The model under review builds one solid part; all positions refer to its coordinate system, in mm. Face numbers are marked on the shaded views. A direction names the side the tool comes from. Coordinates: 2 decimals unless noted, no trailing zeros. Write each loop counter-clockwise with the first axis right and the second up, starting at its lowest first coordinate (ties: lowest second). Pieces come first, ordered by that corner, then holes. Notation, with made-up numbers: (79.5, -37.5) -> (109.5, -37.5) arc R16 ccw to (109.5, -24.5) -> close; hole circle Ø4 at (14.5, 6). An arc over 180 degrees is marked (long way). Write each question's results on one line, items separated by ' | '.
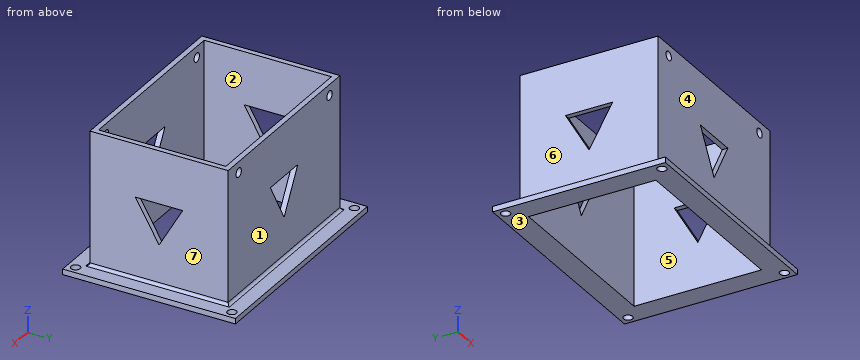
```python
from build123d import *

# Parameters (mm, degrees)
SKETCH_1_W          = 125
SKETCH_1_H          = 95
SKETCH_1_W_2        = 100
SKETCH_1_H_2        = 70
EXTRUDE_1_DEPTH     = 3
SKETCH_2_W          = 106
SKETCH_2_H          = 76
SKETCH_2_W_2        = 100
SKETCH_2_H_2        = 70
EXTRUDE_2_DEPTH     = 73.5
SKETCH_3_R          = 2.5
CUT_EXTRUDE_1_DEPTH = 113.5
FILLET_1_R          = 1.5
SKETCH_4_R          = 2.5
CUT_EXTRUDE_2_DEPTH = 113.5
CUT_EXTRUDE_3_DEPTH = 113.5
CUT_EXTRUDE_4_DEPTH = 113.5


with BuildPart() as part:
    # 草图1 → 凸台-拉伸1 (new body)
    with BuildSketch(Plane.XY):
        Rectangle(SKETCH_1_W, SKETCH_1_H)
        Rectangle(SKETCH_1_W_2, SKETCH_1_H_2, mode=Mode.SUBTRACT)
    extrude(amount=EXTRUDE_1_DEPTH)

    # 草图2 → 凸台-拉伸2 (add)
    with BuildSketch(Plane.XY.offset(3)):
        Rectangle(SKETCH_2_W, SKETCH_2_H)
        Rectangle(SKETCH_2_W_2, SKETCH_2_H_2, mode=Mode.SUBTRACT)
    extrude(amount=EXTRUDE_2_DEPTH)

    # 草图3 → 切除-拉伸1 (cut)
    with BuildSketch(Plane.XZ.offset(38)):
        with Locations(Location((-43, 70.5, 0), (0, 0, 270))):
            Circle(SKETCH_3_R)
        with Locations(Location((43, 70.5, 0), (0, 0, 90))):
            Circle(SKETCH_3_R)
    extrude(amount=-CUT_EXTRUDE_1_DEPTH, mode=Mode.SUBTRACT)

    # 圆角1
    fillet_1_edges = [part.edges().sort_by_distance(p)[0] for p in [
        (53, 0, 3),
        (0, 38, 3),
        (-53, 0, 3),
        (0, -38, 3),
    ]]
    fillet(fillet_1_edges, radius=FILLET_1_R)

    # 草图4 → 切除-拉伸2 (cut)
    with BuildSketch(Plane.XY.offset(3)):
        with Locations((-58, 43)):
            Circle(SKETCH_4_R)
        with Locations((58, 43)):
            Circle(SKETCH_4_R)
        with Locations((58, -43)):
            Circle(SKETCH_4_R)
        with Locations((-58, -43)):
            Circle(SKETCH_4_R)
    extrude(amount=-CUT_EXTRUDE_2_DEPTH, mode=Mode.SUBTRACT)

    # 草图5 → 切除-拉伸3 (cut)
    with BuildSketch(Plane.XZ.offset(38)):
        Polygon((0, 25), (12.990381057, 47.5), (-12.990381057, 47.5), align=None)
    extrude(amount=-CUT_EXTRUDE_3_DEPTH, mode=Mode.SUBTRACT)

    # 草图6 → 切除-拉伸4 (cut)
    with BuildSketch(Plane.ZY.offset(53)):
        Polygon((25, 0), (47.5, -12.990381057), (47.5, 12.990381057), align=None)
    extrude(amount=-CUT_EXTRUDE_4_DEPTH, mode=Mode.SUBTRACT)


solid = part.part
```
Q1. Add section C-C (y = 43). Write out the cut boundary in (x, z), plus the area to 3 significant figures.
Solution:
outline: (-62.5, 0) -> (-60.5, 0) -> (-60.5, 3) -> (-62.5, 3) -> close; (-55.5, 0) -> (55.5, 0) -> (55.5, 3) -> (-55.5, 3) -> close; (60.5, 0) -> (62.5, 0) -> (62.5, 3) -> (60.5, 3) -> close | area: 345 mm²
Q2. Clearance check with flat-ended pins moving along their axes: P1, Ø21, axis at y = -1, z = 20.5, coming from the -X side; P2, Ø1.5, axis at y = 34.5, z = 41, coming from the +X side; P3, Ø3, axis at x = -58, y = -43, coming from the +Z side; P4, Ø4, axis at x = 36, z = 33, coming from the -Y side. State where each tip first meets the part, or that it passes through.
Solution:
P1: x = -53 | P2: x = 53 | P3: through | P4: y = -38
Q3. Add section B-B (z = 70.5). Write out the cut boundary in (x, y).
Solution:
outline: (-53, -38) -> (-45.5, -38) -> (-45.5, -35) -> (-50, -35) -> (-50, 35) -> (-45.5, 35) -> (-45.5, 38) -> (-53, 38) -> close; (-40.5, -38) -> (40.5, -38) -> (40.5, -35) -> (-40.5, -35) -> close; (-40.5, 35) -> (40.5, 35) -> (40.5, 38) -> (-40.5, 38) -> close; (45.5, -38) -> (53, -38) -> (53, 38) -> (45.5, 38) -> (45.5, 35) -> (50, 35) -> (50, -35) -> (45.5, -35) -> close
Q4. Add section D-D (x = 38). Write out the cut boundary in (y, z), plus the area to 3 significant figures.
Solution:
outline: (-47.5, 0) -> (-35, 0) -> (-35, 76.5) -> (-38, 76.5) -> (-38, 4.5) arc R1.5 cw to (-39.5, 3) -> (-47.5, 3) -> close; (35, 0) -> (47.5, 0) -> (47.5, 3) -> (39.5, 3) arc R1.5 cw to (38, 4.5) -> (38, 76.5) -> (35, 76.5) -> close | area: 517 mm²
Q5. For line 1 (X direction, y = -36.65, z = 70.5); line 2 (Y direction, x = -58, z = 2.3); line 3 (Y direction, x = 3, z = 11.5), list the stretches that pass through material, from the lowest coordinate up. Write a range as from..to.
Solution:
line 1: -53..-45.5, -40.5..40.5, 45.5..53 | line 2: -47.5..-45.5, -40.5..40.5, 45.5..47.5 | line 3: -38..-35, 35..38
Q6. Draft analysis for pull direction Y (two halves, no side actions). For the marked faces 1, 2 and 3, state which applies: pulls with the +Y half, pulls with the -Y half, needs draft (parallel to the pull), parting line crosses it, or undercut.
Solution:
face 1: pulls with the +Y half | face 2: undercut | face 3: needs draft
Q7. Machinability: for the marked faces 4, 5, 6 and 7, which of the approach directions +Z, -Z, +X, -X, +Y, -Y give a long, thin tool a straight path to every point of the face, cutting with its end or side? Answer none if there is none.
Solution:
face 4: +Z, +X, -X, -Y | face 5: +Z, -Z | face 6: +Z, -X, +Y, -Y | face 7: +Z, +X, +Y, -Y
Q8. Add section A-A (x = 58). Write out the cut boundary in (y, z).
Solution:
outline: (-47.5, 0) -> (-45.5, 0) -> (-45.5, 3) -> (-47.5, 3) -> close; (-40.5, 0) -> (40.5, 0) -> (40.5, 3) -> (-40.5, 3) -> close; (45.5, 0) -> (47.5, 0) -> (47.5, 3) -> (45.5, 3) -> close
